Can you work these out from the model? Positions are in its coordinate system, mm. A direction names the side the tool comes from. Coordinates: 2 decimals unless noted, no trailing zeros. Order: outer loops, then holes, each group sorted by start corner. A loop starts at its lowest first (then second) coordinate and runs counter-clockwise, first axis right, second up. Notation, with made-up numbers: (-0.5, 32) - (15.5, 32) arc R15 ccw to (15.5, 51) - close; hole circle Ø6 at (31, 28.5). An arc over 180 degrees is marked (long way). Return JSON: item names as keys, results as strings. Group by question number.
1) If we mould it in two halves opening along X, with no side actions, what happens to faces 1 (the face through (0, 51, 26)), 2 (the face through (22, 49, 26)), 3 (the face through (15.55, 44.2, 25.78)), 4 (the face through (-22, 49, 26))? For each: pulls with the +X half, pulls with the -X half, needs draft (parallel to the pull), parting line crosses it, or undercut.
2) If I drill on line 1 along X through (y, z) = (1.5, 0); line 2 along X through (y, z) = (5, 8); line 3 along X through (y, z) = (1.25, -15.5), over which ranges is the centre line in solid material (lowest first)?
3) Imagine slicing it at D-D (z = 0). Write out the boundary of the cut face in (x, y).
4) Imagine slicing it at B-B (z = 15.5). Write out the boundary of the cut face in (x, y), and give its area (3 significant figures).
5) For pin 1 Ø10 at (x, z) = (-16.5, 17.5) entering from +Y; pin 2 Ø3 at (x, y) = (8, 11) entering from -Z, each with a flat end and sliding along its axis, tell me the tip position at first contact or that it passes through.
6) Imagine slicing it at C-C (x = 0). Write out the boundary of the cut face in (y, z).
7) Which directions (+Z, -Z, +X, -X, +Y, -Y) give clear straight access to the entire face, cutting with the end or side of a thin tool? Please do faces 5 (the face through (-0.3, 2.6, -11.3)), 6 (the face through (-15.55, 44.2, 25.78)), 7 (the face through (-22.5, 1.3, -22)).
8) Imagine slicing it at A-A (y = 37). Write out the boundary of the cut face in (x, z), and give its area (3 significant figures).
```python
from build123d import *

# Parameters (mm, degrees)
SKETCH1_W           = 50
SKETCH1_H           = 49
SKETCH1_R           = 1.7
SKETCH1_R_2         = 11
BOSS_EXTRUDE1_DEPTH = 2.6
SKETCH2_W           = 50
SKETCH2_H           = 51
BOSS_EXTRUDE2_DEPTH = 2.6
BOSS_EXTRUDE3_DEPTH = 2.6
CHAMFER1_SIZE       = 5
CHAMFER2_SIZE       = 0.4


with BuildPart() as part:
    # Sketch1 → Boss-Extrude1 (new body)
    with BuildSketch(Plane(origin=(0, 0, 0), x_dir=(1, 0, 0), z_dir=(0, 1, 0))):
        Rectangle(SKETCH1_W, SKETCH1_H)
        with Locations(Location((-15.816326531, 15.5, 0), (0, 0, 270))):
            Circle(SKETCH1_R, mode=Mode.SUBTRACT)
        with Locations(Location((15.816326531, 15.5, 0), (0, 0, 270))):
            Circle(SKETCH1_R, mode=Mode.SUBTRACT)
        with Locations(Location((-15.816326531, -15.5, 0), (0, 0, 270))):
            Circle(SKETCH1_R, mode=Mode.SUBTRACT)
        with Locations(Location((15.816326531, -15.5, 0), (0, 0, 270))):
            Circle(SKETCH1_R, mode=Mode.SUBTRACT)
        with Locations(Location((0, 0, 0), (0, 0, 270))):
            Circle(SKETCH1_R_2, mode=Mode.SUBTRACT)
    extrude(amount=BOSS_EXTRUDE1_DEPTH)

    # Sketch2 → Boss-Extrude2 (add)
    with BuildSketch(Plane.XY.offset(24.5)):
        with Locations((0, 25.5)):
            Rectangle(SKETCH2_W, SKETCH2_H)
        with BuildLine():
            Line((-13.1, 41.8), (-13.1, 11.8))
            ThreePointArc((-13.1, 11.8), (-15.5, 9.4), (-17.9, 11.8))
            Line((-17.9, 11.8), (-17.9, 41.8))
            ThreePointArc((-17.9, 41.8), (-15.5, 44.2), (-13.1, 41.8))
        make_face(mode=Mode.SUBTRACT)
        with BuildLine():
            Line((13.1, 41.8), (13.1, 11.8))
            ThreePointArc((13.1, 11.8), (15.5, 9.4), (17.9, 11.8))
            Line((17.9, 11.8), (17.9, 41.8))
            ThreePointArc((17.9, 41.8), (15.5, 44.2), (13.1, 41.8))
        make_face(mode=Mode.SUBTRACT)
    extrude(amount=BOSS_EXTRUDE2_DEPTH)

    # Sketch3 → Boss-Extrude3 (add)
    with BuildSketch(Plane.ZY.offset(25)):
        Polygon((4.5, 2.6), (24.5, 22.6), (24.5, 2.6), align=None)
    boss_extrude3 = extrude(amount=-BOSS_EXTRUDE3_DEPTH)

    # Mirror1: Boss-Extrude3 across plane
    add(boss_extrude3.mirror(Plane(origin=(0, 0, 0), x_dir=(0, 0, 1), z_dir=(1, 0, 0))))

    # Chamfer1
    chamfer1_edges = [part.edges().sort_by_distance(p)[0] for p in [
        (-25, 51, 25.8),
        (25, 51, 25.8),
        (-25, 1.3, -24.5),
        (25, 1.3, -24.5),
    ]]
    chamfer(chamfer1_edges, length=CHAMFER1_SIZE)

    # Chamfer2
    chamfer2_edges = [part.edges().sort_by_distance(p)[0] for p in [
        (0, 2.6, 24.5),
    ]]
    chamfer(chamfer2_edges, length=CHAMFER2_SIZE)


solid = part.part
```
Calculated:
{
 "1": {"face 1": "needs draft", "face 2": "pulls with the +X half", "face 3": "undercut", "face 4": "pulls with the -X half"},
 "2": {"line 1": "-25 to -11, 11 to 25", "line 2": "-25 to -22.4, 22.4 to 25", "line 3": "-25 to -17.52, -14.12 to 14.12, 17.52 to 25"},
 "3": {"outline": "(-25, 0) - (-11, 0) - (-11, 2.6) - (-25, 2.6) - close; (11, 0) - (25, 0) - (25, 2.6) - (11, 2.6) - close"},
 "4": {"outline": "(-25, 0) - (-17.52, 0) - (-17.52, 2.6) - (-22.4, 2.6) - (-22.4, 13.6) - (-25, 13.6) - close; (-14.12, 0) - (14.12, 0) - (14.12, 2.6) - (-14.12, 2.6) - close; (17.52, 0) - (25, 0) - (25, 13.6) - (22.4, 13.6) - (22.4, 2.6) - (17.52, 2.6) - close", "area": "170 mm2"},
 "5": {"pin 1": "y = 2.6", "pin 2": "z = 24.5"},
 "6": {"outline": "(0, -24.5) - (2.6, -24.5) - (2.6, -11) - (0, -11) - close; (0, 11) - (2.6, 11) - (2.6, 24.1) - (3, 24.5) - (51, 24.5) - (51, 27.1) - (0, 27.1) - close"},
 "7": {"face 5": "-Z, +Y", "face 6": "+Z, -Z", "face 7": "-Z, -X, +Y, -Y"},
 "8": {"outline": "(-25, 24.5) - (-17.9, 24.5) - (-17.9, 27.1) - (-25, 27.1) - close; (-13.1, 24.5) - (13.1, 24.5) - (13.1, 27.1) - (-13.1, 27.1) - close; (17.9, 24.5) - (25, 24.5) - (25, 27.1) - (17.9, 27.1) - close", "area": "105 mm2"}
}
